The listing builds one solid part. Answer for the finished solid, in the listing's coordinates (mm). Face numbers are marked on the shaded views. A direction names the side the tool comes from. Coordinates: 2 decimals unless noted, no trailing zeros. Order: outer loops, then holes, each group sorted by start corner. A loop starts at its lowest first (then second) coordinate and runs counter-clockwise, first axis right, second up.
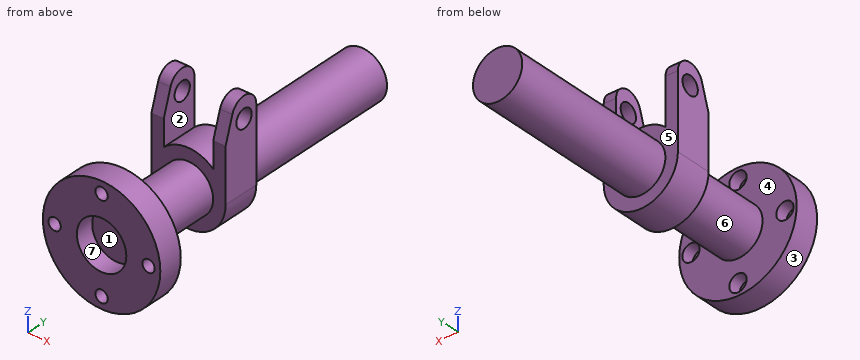
```python
from build123d import *

# Parameters (mm, degrees)
SKETCH2_W           = 10
SKETCH2_H           = 80
BOSS_EXTRUDE1_DEPTH = 30
SKETCH3_R           = 7.5
CUT_EXTRUDE1_DEPTH  = 94
HOLE1_D             = 10
HOLE1_CBORE_D       = 14
HOLE1_CBORE_DEPTH   = 10
SKETCH8_R           = 20
CUT_EXTRUDE2_DEPTH  = 15


with BuildPart() as part:
    # Sketch1 → Revolve1 (revolve)
    with BuildSketch(Plane.XY):
        Polygon((0, 0), (47.5, 0), (47.5, 20), (19.9, 20), (19.9, 85), (30, 85), (30, 115), (19.9, 115), (19.9, 255), (0, 255), align=None)
    revolve(axis=Axis((0, 307.026159996, 0), (0, -1, 0)))

    # Sketch2 → Boss-Extrude1 (add)
    with BuildSketch(Plane(origin=(0, 85, 0), x_dir=(1, 0, 0), z_dir=(0, 1, 0))):
        with Locations((-25, -40)):
            Rectangle(SKETCH2_W, SKETCH2_H)
        with Locations((25, -40)):
            Rectangle(SKETCH2_W, SKETCH2_H)
    extrude(amount=BOSS_EXTRUDE1_DEPTH)

    # Sketch3 → Cut-Extrude1 (cut)
    with BuildSketch(Plane.ZY.offset(30)):
        with Locations((55, 103)):
            Circle(SKETCH3_R)
        with BuildLine():
            Line((43.44222057, 85), (63.709479612, 91.587736377))
            ThreePointArc((63.709479612, 91.587736377), (71.852155152, 104.877875997), (60, 115))
            Line((60, 115), (80, 115))
            Line((80, 115), (80, 85))
            Line((80, 85), (43.44222057, 85))
        make_face()
    extrude(amount=-CUT_EXTRUDE1_DEPTH, mode=Mode.SUBTRACT)

    # Hole1 (through all)
    with Locations(Plane(origin=(0, 20, 0), x_dir=(1, 0, 0), z_dir=(0, 1, 0))):
        with Locations((38, 0), (0, 38), (-38, 0), (0, -38)):
            CounterBoreHole(HOLE1_D / 2, HOLE1_CBORE_D / 2, HOLE1_CBORE_DEPTH)

    # Sketch8 → Cut-Extrude2 (cut)
    with BuildSketch(Plane.XZ):
        Circle(SKETCH8_R)
    extrude(amount=-CUT_EXTRUDE2_DEPTH, mode=Mode.SUBTRACT)


solid = part.part
```
1) Straight lines are drawn through the part: probe 1 along Z at (x, y) = (0, 3.25); probe 2 along Y at (x, z) = (21.5, 12); probe 3 along Y at (x, z) = (-30.5, -32). For each, find the intervals that lie inside material, in ascending order.
2) For the marked faces 5, 6 and 7, determine the directions among +Z, -Z, +X, -X, +Y, -Y from which every point of the face is accessible in a straight line to the end or side of a thin tool.
3) Each of these flat-tipped pins is pushed along its axis until it touches: P1, Ø12, axis at y = 116, z = 37.5, coming from the +X side; P2, Ø9, axis at y = 103, z = 55, coming from the -X side; P3, Ø13, axis at x = 0, z = -38, coming from the +Y side; P4, Ø1.5, axis at x = 29, z = 41, coming from the +Y side. Where does it stop, or does it pass through?
4) A cutting plane is placed at B-B, the plane z = -38. Write down the section's boundary in (x, y).
5) The mould has two halves that part along X. Classify the marked faces 1, 2, 3 and 4: released by +X, released by -X, zero draft, split by the parting line, or undercut.
6) A cutting plane is placed at A-A, the plane z = 38. Write down the section's boundary in (x, y), plus the area to 3 significant figures.
7) A cutting plane is placed at C-C, the plane x = -38. Write down the section's boundary in (y, z).
8) A cutting plane is placed at D-D, the plane x = 0. Count the separate pieces of the cut face and the enclosed holes in it, plus the area to 3 significant figures.
Working result:
1. probe 1: z = -47.5 to -43, -33 to -20, 20 to 33, 43 to 47.5
1. probe 2: y = 0 to 20, 85 to 115
1. probe 3: y = 0 to 20
2. face 5: +Y
2. face 6: none
2. face 7: -Y
3. P1: stops at x = 30
3. P2: passes through
3. P3: stops at y = 10
3. P4: stops at y = 115
4. outline: (-28.5, 0) - (-5, 0) - (-5, 10) - (-7, 10) - (-7, 20) - (-28.5, 20) - close; (5, 0) - (28.5, 0) - (28.5, 20) - (7, 20) - (7, 10) - (5, 10) - close
5. face 1: undercut
5. face 2: undercut
5. face 3: split by the parting line
5. face 4: zero draft
6. outline: (-30, 85) - (-20, 85) - (-20, 115) - (-30, 115) - close; (-28.5, 0) - (-5, 0) - (-5, 10) - (-7, 10) - (-7, 20) - (-28.5, 20) - close; (5, 0) - (28.5, 0) - (28.5, 20) - (7, 20) - (7, 10) - (5, 10) - close; (20, 85) - (30, 85) - (30, 115) - (20, 115) - close
6. area: 1,500 mm2
7. outline: (0, -28.5) - (20, -28.5) - (20, -7) - (10, -7) - (10, -5) - (0, -5) - close; (0, 5) - (10, 5) - (10, 7) - (20, 7) - (20, 28.5) - (0, 28.5) - close
8. separate pieces: 3
8. enclosed holes: 0
8. area: 10,800 mm2
